from build123d import *

# Parameters (mm, degrees)
F0_R     = 100
F1_DEPTH = 7
F2_R     = 11
F3_DEPTH = 25


with BuildPart() as f1:
    # F0 (on Top) → F1 (new body)
    with BuildSketch(Plane.XY):
        Circle(F0_R)
    extrude(amount=F1_DEPTH)

    # F2 (on Top) → F3 (cut)
    with BuildSketch(Plane.XY):
        Circle(F2_R)
        with Locations((0, 57.71517)):
            Circle(F2_R)
        with Locations((-49.982803, -28.857585)):
            Circle(F2_R)
        with Locations((49.982803, -28.857585)):
            Circle(F2_R)
    extrude(amount=F3_DEPTH, mode=Mode.SUBTRACT)


solid = f1.part
Input: part model. Units: mm. Frame: model coordinates. Coordinates: 2 decimals unless noted, no trailing zeros. Loops run counter-clockwise (first coordinate to the right, second up) from the corner with the lowest first, then second, coordinate; pieces in that order, holes last.
Q1. Cut plane B-B (x = 0). Output: boundary loops of the cut face in (y, z), then the cut area to 3 significant figures.
Q2. Draft query along Y for faces 1 (the face through (95.38, 30.04, 3.45)), 2 (the face through (-1, -21, 7)), 3 (the face through (-39.82, -33.07, 3.45)). Return one class per face: +Y half, -Y half, draft (parallel to the pull), parting line (faces both ways), or undercut.
Q3. Cut plane C-C (x = -45.5). Output: boundary loops of the cut face in (y, z).
Q4. Cut plane A-A (y = 0). Output: boundary loops of the cut face in (x, z), then the cut area to 3 significant figures.
Q5. Cut plane D-D (y = -26). Output: boundary loops of the cut face in (x, z).
Q6. Material intervals for line 1 (Y direction, x = 0, z = 4); line 2 (Y direction, x = 2, z = 6.5); line 3 (X direction, y = -34.5, z = 3), sorted ascending.
Q7. Contact query for flat-ended pins moving along their axis: pin 1 (4 mm diameter, centred on y = 61, z = 5.5, fed in from +X); pin 2 (6 mm diameter, centred on x = 30, y = -23, fed in from -Z); pin 3 (1.5 mm diameter, centred on y = 68.5, z = 2.5, fed in from -X); pin 4 (1 mm diameter, centred on y = -22, z = 5.5, fed in from +X). Output: stop coordinate, or through.
Working result:
1. outline: (-100, 0) - (-11, 0) - (-11, 7) - (-100, 7) - close; (11, 0) - (46.72, 0) - (46.72, 7) - (11, 7) - close; (68.72, 0) - (100, 0) - (100, 7) - (68.72, 7) - close
1. area: 1,090 mm2
2. face 1: parting line
2. face 2: draft
2. face 3: undercut
3. outline: (-89.05, 0) - (-38.9, 0) - (-38.9, 7) - (-89.05, 7) - close; (-18.81, 0) - (89.05, 0) - (89.05, 7) - (-18.81, 7) - close
4. outline: (-100, 0) - (-11, 0) - (-11, 7) - (-100, 7) - close; (11, 0) - (100, 0) - (100, 7) - (11, 7) - close
4. area: 1,250 mm2
5. outline: (-96.56, 0) - (-60.61, 0) - (-60.61, 7) - (-96.56, 7) - close; (-39.36, 0) - (39.36, 0) - (39.36, 7) - (-39.36, 7) - close; (60.61, 0) - (96.56, 0) - (96.56, 7) - (60.61, 7) - close
6. line 1: y = -100 to -11, 11 to 46.72, 68.72 to 100
6. line 2: y = -99.98 to -10.82, 10.82 to 46.9, 68.53 to 99.98
6. line 3: x = -93.86 to -59.43, -40.54 to 40.54, 59.43 to 93.86
7. pin 1: stops at x = 80.74
7. pin 2: stops at z = 0
7. pin 3: stops at x = -73.55
7. pin 4: stops at x = 97.66
